Could you check a few things on this model? Use its own coordinates, in mm. A direction names the side the tool comes from. Round coordinates to 2 decimals unless told otherwise and drop trailing zeros. Loops run counter-clockwise (first coordinate to the right, second up) from the corner with the lowest first, then second, coordinate; pieces in that order, holes last.
Autodesk Inventor part; units mm, degrees
ref_plane "YZ Plane" through (0, 0, 0) normal (1, 0, 0) x (0, 1, 0)
ref_plane "XZ Plane" through (0, 0, 0) normal (0, 1, 0) x (-1, 0, 0)
ref_plane "XY Plane" through (0, 0, 0) normal (0, 0, 1) x (1, 0, 0)
sketch "Sketch1" plane through (0, 0, 0) normal (0, 1, 0) x (-1, 0, 0)
  line L0 (-51.65, 23.5) -> (51.65, 23.5)
  line L1 (54.65, 20.5) -> (54.65, -20.5)
  line L2 (51.65, -23.5) -> (-51.65, -23.5)
  line L3 (-54.65, -20.5) -> (-54.65, 20.5)
  circle A0 centre (-47.65, 16.5) radius 2.25
  circle A1 centre (47.65, 16.5) radius 2.25
  circle A2 centre (-47.65, 16.5) radius 26.75 construction
  circle A3 centre (-10.7, 16.5) radius 2.25
  circle A4 centre (-10.7, 16.5) radius 11.2 construction
  line L4 (-21.9, 16.5) -> (-21.9, 6.8604)
  line L5 (-20.9, 16.5) -> (-20.9, 6.8604)
  circle A5 centre (10.7, 16.5) radius 2.25
  circle A6 centre (10.7, 16.5) radius 11.2 construction
  line L6 (-0.5, 16.5) -> (-0.5, 5.694)
  line L7 (0.5, 16.5) -> (0.5, 5.694)
  circle A7 centre (47.65, 16.5) radius 26.75 construction
  line L8 (20.9, 16.5) -> (20.9, 5.8426)
  line L9 (21.9, 16.5) -> (21.9, 5.8426)
  arc A8 (-51.65, 23.5) -> (-54.65, 20.5) centre (-51.65, 20.5) ccw
  arc A9 (-54.65, -20.5) -> (-51.65, -23.5) centre (-51.65, -20.5) ccw
  arc A10 (54.65, 20.5) -> (51.65, 23.5) centre (51.65, 20.5) ccw
  arc A11 (51.65, -23.5) -> (54.65, -20.5) centre (51.65, -20.5) ccw
  line L10 (-84.9483, 16.5) -> (77.5332, 16.5) construction
  line L11 (-54.65, 0) -> (54.65, 0)
  line L12 (10.7, 30.5) -> (10.7, -33.5) construction
  circle A12 centre (10.7, -16.5) radius 2.25
  line L13 (5, -8.5) -> (18, -8.5) construction
  line L14 (3.7, -4.5) -> (3.7, -33.5) construction
  line L15 (-6.3, -4.5) -> (-6.3, -33.5) construction
  line L16 (-1.3, -33.5) -> (-1.3, -4.5) construction
  circle A13 centre (-1.3, -38.9) radius 2.25
  circle A14 centre (-1.3, -8.5) radius 2.25
  line L17 (-17.7373, -23.5) -> (14.2274, -23.5)
  line L18 (14.2274, -23.5) -> (14.2274, -45.3565)
  line L19 (14.2274, -45.3565) -> (-17.7373, -45.3565)
  line L20 (-17.7373, -45.3565) -> (-17.7373, -23.5)
  line L21 (-40.65, 5) -> (-30.65, 5)
  line L22 (-30.65, 5) -> (-30.65, -5)
  line L23 (-30.65, -5) -> (-40.65, -5)
  line L24 (-40.65, -5) -> (-40.65, 5)
  line L25 (-42.65, -7) -> (-28.65, -7)
  line L26 (-28.65, -7) -> (-28.65, 7)
  line L27 (-28.65, 7) -> (-42.65, 7)
  line L28 (-42.65, 7) -> (-42.65, -7)
  point P0 (0, 0)
  point P1 (-54.65, 23.5)
  point P2 (-54.65, -23.5)
  point P3 (0, 23.5)
  point P4 (-35.65, 5)
  point P5 (-30.65, 0)
  dimension "d5" = 53.5
  dimension "d12" = 53.5
  dimension "d1" = 4.5
  dimension "d2" = 7
  dimension "d3" = 4.5
  dimension "d4" = 7
  dimension "d6" = 4.5
  dimension "d7" = 22.4
  dimension "d8" = 1
  dimension "d9" = 4.5
  dimension "d10" = 22.4
  dimension "d11" = 1
  dimension "d13" = 1
  dimension "d14" = 3
  dimension "d23" = 16.5
  dimension "d24" = 7
  dimension "d27" = 8
  dimension "d28" = 7
  dimension "d29" = 10
  dimension "d30" = 5
  dimension "d31" = 4.5
  dimension "d32" = 4.5
  dimension "d33" = 30.4
  dimension "d38" = 0
  dimension "d40" = 10
  dimension "d41" = 10
  dimension "d43" = 2
  dimension "d47" = 12
extrude "Extrusion1" add sketch "Sketch1" along normal blind 3 contours L0 A10 L1 L11 L26 L27 L28 L3 A8 | L11 L28 L25 L26 L1 A11 L2 A9 L3 | L28 L27 L26 L11 L22 L21 L24 | L11 L24 L23 L22 L26 L25 L28 | L24 L21 L22 L11 | L11 L22 L23 L24 | A0 | A1 | A3 | A5 | A12 | A14
extrude "Extrusion2" cut sketch "Sketch1" along normal blind 10 contours A0 | A1 | A3 | A5
mirror "Mirror1" about plane through (0, 0, 0) normal (0, 0, 1) of "Extrusion2"
extrude "Extrusion3" add sketch "Sketch1" along normal blind 3 contours L2 L18 L19 L20
extrude "Extrusion4" cut sketch "Sketch1" along normal blind 3 contours A14
fillet "Fillet1" radius 3 2 edges at (-14.2274, 1.5, -45.3565) (17.7373, 1.5, -45.3565)
extrude "Extrusion5" cut sketch "Sketch1" along normal blind 1 contours L28 L27 L26 L11 L22 L21 L24 | L11 L24 L23 L22 L26 L25 L28
mirror "Mirror2" about plane through (0, 0, 0) normal (1, 0, 0) of "Extrusion5"
properties part number "OuterBar"
Item 1: If we section it at D-D, the plane x = 1.3: Please give me the cut outline in (y, z).
Results list:
outline: (0, -45.36) - (3, -45.36) - (3, -41.15) - (0, -41.15) - close; (0, -36.65) - (3, -36.65) - (3, -10.75) - (0, -10.75) - close; (0, -6.25) - (3, -6.25) - (3, 23.5) - (0, 23.5) - close
Item 2: If we section it at A-A, the plane z = 16.5: Please give me the cut outline in (x, y).
Results list:
outline: (-54.65, 0) - (-49.9, 0) - (-49.9, 3) - (-54.65, 3) - close; (-45.4, 0) - (-12.95, 0) - (-12.95, 3) - (-45.4, 3) - close; (-8.45, 0) - (8.45, 0) - (8.45, 3) - (-8.45, 3) - close; (12.95, 0) - (45.4, 0) - (45.4, 3) - (12.95, 3) - close; (49.9, 0) - (54.65, 0) - (54.65, 3) - (49.9, 3) - close
Item 3: Will these pins go through, and if not, where does the flat tip stop? pin 1 (1.5 mm diameter, centred on x = 35.5, y = 1, fed in from -Z); pin 2 (4 mm diameter, centred on x = -10.7, z = -16.5, fed in from +Y).
Results list:
pin 1: stops at z = -23.5
pin 2: passes through
Item 4: We'd pull the mould along Z, two halves only. Please class faces 3 (the flat face through (17.737, 1, -33)), 4 (the cylindrical face through (-13.325, 1.521, -44.501)), 5 (the cylindrical face through (48.138, 1.479, -14.304)): released by +Z, released by -Z, zero draft, split by the parting line, or undercut.
Results list:
face 3: zero draft
face 4: released by -Z
face 5: undercut
Item 5: For faces 1 (the flat face through (-33, 1, -23.5)), 2 (the cylindrical face through (-10.212, 1.479, 18.696)), which set-ups out of +Z, -Z, +X, -X, +Y, -Y let a thin tool reach every point of the face, with its end or its side?
Results list:
face 1: -Z, -X, +Y, -Y
face 2: +Y, -Y
Item 6: If I drill on line 1 along X through (y, z) = (0.9, -16.5); line 2 along Z through (x, y) = (10.7, 0.85); line 3 along Z through (x, y) = (47.65, 1.1), over which ranges is the centre line in solid material (lowest first)?
Results list:
line 1: x = -54.65 to -49.9, -45.4 to -12.95, -8.45 to 8.45, 12.95 to 45.4, 49.9 to 54.65
line 2: z = -45.36 to -18.75, -14.25 to 14.25, 18.75 to 23.5
line 3: z = -23.5 to -18.75, -14.25 to 14.25, 18.75 to 23.5
Item 7: If we section it at C-C, the plane z = -8.5: Please give me the cut outline in (x, y), then the cut area to 3 significant figures.
Results list:
outline: (-54.65, 0) - (-0.95, 0) - (-0.95, 3) - (-54.65, 3) - close; (3.55, 0) - (54.65, 0) - (54.65, 3) - (3.55, 3) - close
area: 314 mm2
Item 8: If we section it at B-B, the plane y = 2.25: Count the separate pieces of the cut face and the enclosed holes in it, then the cut area to 3 significant figures.
Results list:
separate pieces: 1
enclosed holes: 10
area: 5,670 mm2
